The model under review builds one solid part; all positions refer to its coordinate system, in mm. A direction names the side the tool comes from. Coordinates: 2 decimals unless noted, no trailing zeros. Write each loop counter-clockwise with the first axis right and the second up, starting at its lowest first coordinate (ties: lowest second). Pieces come first, ordered by that corner, then holes. Notation, with made-up numbers: (9.25, 69) -> (35.25, 69) arc R11 ccw to (35.25, 88) -> close; hole circle Ø10 at (-30, 11.5). An arc over 180 degrees is marked (long way). Write each question's results on one line, items separated by ' | '.
```python
from build123d import *

# Parameters (mm, degrees)
PAD_DEPTH       = 6
POCKET_DEPTH    = 3
SKETCH002_W     = 18.4
SKETCH002_H     = 20.85
POCKET001_DEPTH = 3
SKETCH003_W     = 8
SKETCH003_H     = 1.65
POCKET002_DEPTH = 3
PAD001_DEPTH    = 3
SKETCH005_W     = 170.5
SKETCH005_H     = 5.95
PAD002_DEPTH    = 3
SKETCH007_R     = 0.8
POCKET003_DEPTH = 563.341185
SKETCH008_W     = 4
SKETCH008_H     = 5.84
POCKET004_DEPTH = 3


with BuildPart() as part:
    # Sketch → Pad (new body)
    with BuildSketch(Plane.XY):
        with BuildLine():
            ThreePointArc((-95, 37.5), (-132.5, 0), (-95, -37.5))
            Line((-95, -37.5), (95, -37.5))
            ThreePointArc((95, -37.5), (132.5, 0), (95, 37.5))
            Line((-95, 37.5), (95, 37.5))
        make_face()
    extrude(amount=PAD_DEPTH)

    # Sketch001 (on Face6 of Pad) → Pocket (cut)
    with BuildSketch(Plane.XY.offset(6)):
        with BuildLine():
            ThreePointArc((-87.3, 6), (-93.3, 0), (-87.3, -6))
            Line((-87.3, -6), (87.3, -6))
            ThreePointArc((87.3, -6), (93.3, 0), (87.3, 6))
            Line((-87.3, 6), (87.3, 6))
        make_face()
    extrude(amount=-POCKET_DEPTH, mode=Mode.SUBTRACT)

    # Sketch002 (on Face5 of Pocket) → Pocket001 (cut)
    with BuildSketch(Plane.XY.offset(6)):
        with Locations((0, -25.425)):
            Rectangle(SKETCH002_W, SKETCH002_H)
    extrude(amount=-POCKET001_DEPTH, mode=Mode.SUBTRACT)

    # Sketch003 (on Face5 of Pocket001) → Pocket002 (cut)
    with BuildSketch(Plane.XY.offset(6)):
        with Locations((0, -36.675)):
            Rectangle(SKETCH003_W, SKETCH003_H)
    extrude(amount=-POCKET002_DEPTH, mode=Mode.SUBTRACT)

    # Sketch004 (on Face5 of Pocket002) → Pad001 (join)
    with BuildSketch(Plane.XY.offset(6)):
        with BuildLine():
            ThreePointArc((-95, 37.5), (-132.5, 0), (-95, -37.5))
            Line((-95, -37.5), (95, -37.5))
            ThreePointArc((95, -37.5), (132.5, 0), (95, 37.5))
            Line((-95, 37.5), (95, 37.5))
        make_face()
        with BuildLine():
            ThreePointArc((-87.3, 6), (-93.3, 0), (-87.3, -6))
            Line((-87.3, -6), (87.3, -6))
            ThreePointArc((87.3, -6), (93.3, 0), (87.3, 6))
            Line((-87.3, 6), (87.3, 6))
        make_face(mode=Mode.SUBTRACT)
    extrude(amount=PAD001_DEPTH)

    # Sketch005 (on Face12 of Pad001) → Pad002 (join)
    with BuildSketch(Plane.XY.offset(9)):
        with BuildLine():
            ThreePointArc((-95, 37.5), (-132.5, 0), (-95, -37.5))
            Line((-95, -37.5), (95, -37.5))
            ThreePointArc((95, -37.5), (132.5, 0), (95, 37.5))
            Line((-95, 37.5), (95, 37.5))
        make_face()
        Rectangle(SKETCH005_W, SKETCH005_H, mode=Mode.SUBTRACT)
    extrude(amount=PAD002_DEPTH)

    # Sketch007 (on Face20 of Pad002) → Pocket003 (cut, through all)
    with BuildSketch(Plane.XY.offset(12)):
        with Locations((-90, -8)):
            Circle(SKETCH007_R)
        with Locations((-90, 8)):
            Circle(SKETCH007_R)
        with Locations((-76, 8)):
            Circle(SKETCH007_R)
        with Locations((-76, -8)):
            Circle(SKETCH007_R)
    pocket003 = extrude(amount=-POCKET003_DEPTH, mode=Mode.SUBTRACT)

    # Mirrored: Pocket003 across Sketch007 V_Axis
    add(pocket003.mirror(Plane(origin=(0, 0, 12), x_dir=(0, 0, 1), z_dir=(1, 0, 0))), mode=Mode.SUBTRACT)

    # Sketch008 (on Face5 of Pocket) → Pocket004 (cut)
    with BuildSketch(Plane.XY.offset(6)):
        with Locations((-94.541526, 0)):
            Rectangle(SKETCH008_W, SKETCH008_H)
        with Locations((94.541526, 0)):
            Rectangle(SKETCH008_W, SKETCH008_H)
    extrude(amount=-POCKET004_DEPTH, mode=Mode.SUBTRACT)


solid = part.part
```
Q1. Add section A-A (y = 0). Write out the cut boundary in (x, z).
Solution:
outline: (-132.5, 0) -> (132.5, 0) -> (132.5, 12) -> (85.25, 12) -> (85.25, 9) -> (93.3, 9) -> (93.3, 6) -> (96.54, 6) -> (96.54, 3) -> (-96.54, 3) -> (-96.54, 6) -> (-93.3, 6) -> (-93.3, 9) -> (-85.25, 9) -> (-85.25, 12) -> (-132.5, 12) -> close
Q2. Add section C-C (y = -19). Write out the cut boundary in (x, z).
Solution:
outline: (-127.33, 0) -> (127.33, 0) -> (127.33, 12) -> (-127.33, 12) -> close; hole (-9.2, 3) -> (9.2, 3) -> (9.2, 6) -> (-9.2, 6) -> close
Q3. Add section D-D (y = 13). Write out the cut boundary in (x, z).
Solution:
outline: (-130.17, 0) -> (130.17, 0) -> (130.17, 12) -> (-130.17, 12) -> close
Q4. Machinability: for faces 1 (the flat face through (-2, 9, 12)), 2 (the cylindrical face through (-93.3, 0.1, 6.6)), which of the approach directions +Z, -Z, +X, -X, +Y, -Y give a long, thin tool a straight path to every point of the face, cutting with its end or side? Answer none if there is none.
Solution:
face 1: +Z, +X, -X, +Y, -Y | face 2: none
Q5. Clearance check with flat-ended pins moving along their axes: P1, Ø3.5, axis at y = -0.5, z = 4, coming from the -X side; P2, Ø0.9, axis at y = 0.5, z = 10.5, coming from the +X side. State where each tip first meets the part, or that it passes through.
Solution:
P1: x = -132.5 | P2: x = 132.5
Q6. Add section B-B (x = 55). Write out the cut boundary in (y, z) (3 decimals).
Solution:
outline: (-37.5, 0) -> (37.5, 0) -> (37.5, 12) -> (2.975, 12) -> (2.975, 9) -> (6, 9) -> (6, 3) -> (-6, 3) -> (-6, 9) -> (-2.975, 9) -> (-2.975, 12) -> (-37.5, 12) -> close
Q7. For line 1 (Y direction, x = -76, z = 5.75); line 2 (Y direction, x = -37, z = 10) (3 decimals); line 3 (Y direction, x = 90, z = 7.25), list the stretches that pass through material, from the lowest coordinate up. Write a range as from..to.
Solution:
line 1: -37.5..-8.8, -7.2..-6, 6..7.2, 8.8..37.5 | line 2: -37.5..-2.975, 2.975..37.5 | line 3: -37.5..-8.8, -7.2..-5.36, 5.36..7.2, 8.8..37.5
Q8. Draft analysis for pull direction X (two halves, no side actions). For faces 3 (the flat face through (-1, 4, 9)), 4 (the cylindrical face through (-132.49, 0.82, 5.92)), 5 (the flat face through (0, -26, 6)), 6 (the flat face through (-1, 37.5, 6)), state which applies: pulls with the +X half, pulls with the -X half, needs draft (parallel to the pull), parting line crosses it, or undercut.
Solution:
face 3: undercut | face 4: pulls with the -X half | face 5: undercut | face 6: needs draft
